Autodesk Inventor part; units mm, degrees
ref_plane "YZ Plane" through (0, 0, 0) normal (1, 0, 0) x (0, 1, 0)
ref_plane "XZ Plane" through (0, 0, 0) normal (0, 1, 0) x (-1, 0, 0)
ref_plane "XY Plane" through (0, 0, 0) normal (0, 0, 1) x (1, 0, 0)
sketch "Sketch1" plane through (0, 0, 0) normal (0, 1, 0) x (-1, 0, 0)
  circle A0 centre (0, 0) radius 2.1
  line L0 (0, -3.9007) -> (-2.84, -3.9007)
  line L1 (-5.4993, -8.2) -> (-3.1, -8.2)
  line L2 (-3.1, -8.2) -> (-4.9, -10)
  line L3 (-4.9, -10) -> (-10, -10)
  line L4 (-10, -10) -> (-10, -4.9)
  line L5 (-10, -4.9) -> (-8.2, -3.1)
  line L6 (-8.2, -3.1) -> (-8.2, -5.4993)
  line L7 (-3.9007, -2.84) -> (-3.9007, 0)
  line L8 (-3.9007, 0) -> (-2.1, 0)
  line L9 (0, -3.9007) -> (0, -2.1) construction
  line L10 (-5.4993, -8.2) -> (-5.4993, -6.56)
  line L11 (-5.4993, -6.56) -> (-2.84, -3.9007)
  line L12 (-3.9007, -2.84) -> (-6.56, -5.4993)
  line L13 (-6.56, -5.4993) -> (-8.2, -5.4993)
  line L14 (6.56, -5.4993) -> (3.9007, -2.84)
  line L15 (3.1, -8.2) -> (5.4993, -8.2)
  line L16 (5.4993, -6.56) -> (5.4993, -8.2)
  line L17 (8.2, -5.4993) -> (8.2, -3.1)
  line L18 (8.2, -5.4993) -> (6.56, -5.4993)
  line L19 (8.2, -3.1) -> (10, -4.9)
  line L20 (4.9, -10) -> (3.1, -8.2)
  line L21 (10, -4.9) -> (10, -10)
  line L22 (10, -10) -> (4.9, -10)
  line L23 (2.84, -3.9007) -> (0, -3.9007)
  line L24 (0, -3.9007) -> (0, -2.1) construction
  line L25 (3.9007, 0) -> (2.1, 0)
  line L26 (3.9007, 0) -> (3.9007, -2.84)
  line L27 (2.84, -3.9007) -> (5.4993, -6.56)
  line L28 (5.4993, 6.56) -> (2.84, 3.9007)
  line L29 (8.2, 3.1) -> (8.2, 5.4993)
  line L30 (6.56, 5.4993) -> (8.2, 5.4993)
  line L31 (5.4993, 8.2) -> (3.1, 8.2)
  line L32 (5.4993, 8.2) -> (5.4993, 6.56)
  line L33 (3.1, 8.2) -> (4.9, 10)
  line L34 (10, 4.9) -> (8.2, 3.1)
  line L35 (4.9, 10) -> (10, 10)
  line L36 (10, 10) -> (10, 4.9)
  line L37 (3.9007, 2.84) -> (3.9007, 0)
  line L38 (3.9007, 0) -> (2.1, 0) construction
  line L39 (0, 3.9007) -> (0, 2.1)
  line L40 (0, 3.9007) -> (2.84, 3.9007)
  line L41 (3.9007, 2.84) -> (6.56, 5.4993)
  line L42 (-6.56, 5.4993) -> (-3.9007, 2.84)
  line L43 (-3.1, 8.2) -> (-5.4993, 8.2)
  line L44 (-5.4993, 6.56) -> (-5.4993, 8.2)
  line L45 (-8.2, 5.4993) -> (-8.2, 3.1)
  line L46 (-8.2, 5.4993) -> (-6.56, 5.4993)
  line L47 (-8.2, 3.1) -> (-10, 4.9)
  line L48 (-4.9, 10) -> (-3.1, 8.2)
  line L49 (-10, 4.9) -> (-10, 10)
  line L50 (-10, 10) -> (-4.9, 10)
  line L51 (-2.84, 3.9007) -> (0, 3.9007)
  line L52 (0, 3.9007) -> (0, 2.1) construction
  line L53 (-3.9007, 0) -> (-2.1, 0) construction
  line L54 (-3.9007, 0) -> (-3.9007, 2.84)
  line L55 (-2.84, 3.9007) -> (-5.4993, 6.56)
  point P0 (0, -3.0003)
  point P1 (-3.0003, 0)
  point P2 (0, -3.0003)
  point P3 (3.0003, 0)
  point P4 (3.0003, 0)
  point P5 (0, 3.0003)
  point P6 (0, 3.0003)
  point P7 (-3.0003, 0)
  dimension "d0" = 4.2
  dimension "d2" = 45
  dimension "d3" = 3.1
  dimension "d4" = 2.84
  dimension "d7" = 10
  dimension "d8" = 10
  dimension "d9" = 1.5
  dimension "d10" = 1.8
  dimension "d11" = 1.64
  dimension "d14" = 360
extrude "Extrusion1" add sketch "Sketch1" along normal mid plane 45 contours L25 L26 L14 L18 L17 L19 L21 L22 L20 L15 L16 L27 L23 L0 L11 L10 L1 L2 L3 L4 L5 L6 L13 L12 L7 L8 A0 | A0 L39 L40 L28 L32 L31 L33 L35 L36 L34 L29 L30 L41 L37 L25 | A0 L8 L54 L42 L46 L45 L47 L49 L50 L48 L43 L44 L55 L51 L39
properties part number "vslot_45mm" material "Aluminum 6061-AHC"
Build history of the part. All positions in model axes, mm. A direction names the side the tool comes from. Give positions to 0.01 mm unless a question says otherwise; leave off trailing zeros. Write each loop counter-clockwise with the first axis right and the second up, starting at its lowest first coordinate (ties: lowest second). Pieces come first, ordered by that corner, then holes. Notation, with made-up numbers: (-34, -39) - (0, -39) arc R14 ccw to (0, -27) - close; hole circle Ø3 at (-39, 58). An arc over 180 degrees is marked (long way). Use one line per item in the form item = value. Start each with the question number.
1. Drop flat-ended pins along their axis: pin 1 Ø6 at (x, y) = (-0.5, 8) entering from +Z; pin 2 Ø2 at (y, z) = (-6, -3.5) entering from -X; pin 3 Ø1 at (y, z) = (12, 2) entering from -X; pin 4 Ø1.5 at (x, z) = (-1.5, -6) entering from +Y. Give the stop position or say it passes through.
2. 3-axis set-ups, long thin cutter, end or side, ignore diameter. For faces 4 (the face through (9.1, -0.3, -4)), 5 (the face through (-5.25, -0.32, -4.19)), 6 (the face through (0.1, 22.5, 2.4)): which of +Z, -Z, +X, -X, +Y, -Y reach the whole face in a straight line?
3. Probe line 1 (X direction, y = 1, z = 0); line 2 (X direction, y = 18, z = 6.75). List the from-to ranges inside material, lowest first. Write a range as [from, to].
4. Band-saw the part on A-A on x = 7. Write the cut outline in (y, z), plus the area to 3 significant figures.
5. Band-saw the part on B-B on z = 0. Write the cut outline in (x, y), plus the area to 3 significant figures.
6. Two-plate mould, pull along Z, no slides. Class faces 1 (the face through (4, -0.3, -9.1)), 2 (the face through (5.21, -0.32, -4.15)), 3 (the face through (0, 0, 3.901)): released by +Z, released by -Z, zero draft, split by the parting line, or undercut.
Conclusion:
q1.pin_1 = 8.6
q1.pin_2 = -9.6
q1.pin_3 = -3.9
q1.pin_4 = through
q2.face_4 = +X, +Y, -Y
q2.face_5 = +Y, -Y
q2.face_6 = +Z, -Z, +X, -X, +Y
q3.line_1 = [-3.9, -2.1], [2.1, 3.9]
q3.line_2 = [-10, -5.5], [5.5, 10]
q4.outline = (-22.5, -10) - (22.5, -10) - (22.5, -5.5) - (-22.5, -5.5) - close; (-22.5, 5.5) - (22.5, 5.5) - (22.5, 10) - (-22.5, 10) - close
q4.area = 405 mm²
q5.outline = (-3.9, -22.5) - (-2.1, -22.5) - (-2.1, 22.5) - (-3.9, 22.5) - close; (2.1, -22.5) - (3.9, -22.5) - (3.9, 22.5) - (2.1, 22.5) - close
q5.area = 162 mm²
q6.face_1 = released by -Z
q6.face_2 = undercut
q6.face_3 = released by +Z
